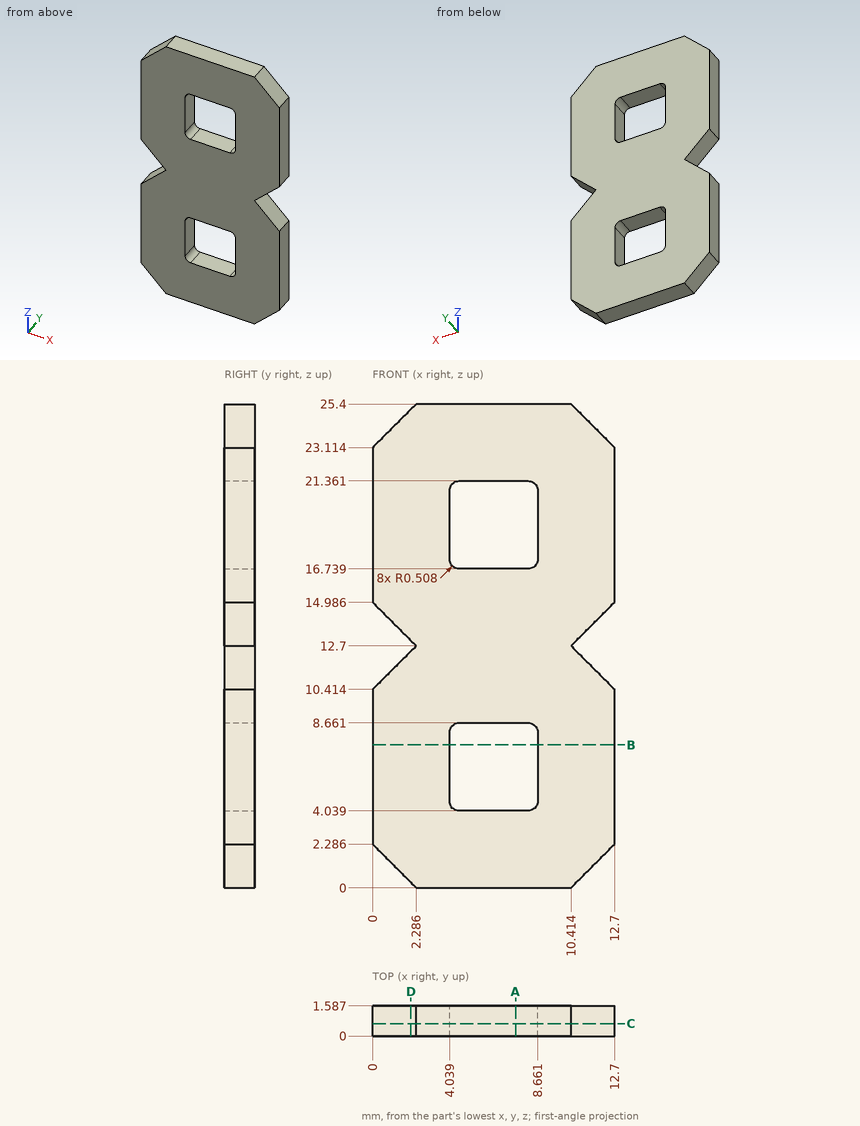
Answer from the drawing. Dimensions are ordinates in mm from the lowest x, y and z of the part. Round coordinates to 2 decimals unless told otherwise and drop trailing zeros. Write each loop counter-clockwise with the first axis right and the second up, starting at its lowest first coordinate (ties: lowest second). Pieces come first, ordered by that corner, then holes.
1. The part is cut by section B-B, the plane z = 7.5. Determine the outline of the cut face in (x, y), then the cut area to 3 significant figures.
2. The part is cut by section C-C, the plane y = 0.65. State how many separate pieces and enclosed holes the cut face has, then the cut area to 3 significant figures.
3. The part is cut by section D-D, the plane x = 2. Determine the outline of the cut face in (y, z) (1 decimal).
4. The part is cut by section A-A, the plane x = 7.5. Determine the outline of the cut face in (y, z).
5. Straight lines are drawn through the part: L1, parallel to Z at x = 7.75, y = 1.4; L2, parallel to X at y = 0.75, z = 7; L3, parallel to Z at x = 12.25, y = 1.1 (1 decimal). For each, find the intervals that lie inside material, in ascending order.
Values:
1. outline: (0, 0) - (4.04, 0) - (4.04, 1.59) - (0, 1.59) - close; (8.66, 0) - (12.7, 0) - (12.7, 1.59) - (8.66, 1.59) - close
1. area: 12.8 mm2
2. separate pieces: 1
2. enclosed holes: 2
2. area: 259 mm2
3. outline: (0, 0.3) - (1.6, 0.3) - (1.6, 12.4) - (0, 12.4) - close; (0, 13) - (1.6, 13) - (1.6, 25.1) - (0, 25.1) - close
4. outline: (0, 0) - (1.59, 0) - (1.59, 4.04) - (0, 4.04) - close; (0, 8.66) - (1.59, 8.66) - (1.59, 16.74) - (0, 16.74) - close; (0, 21.36) - (1.59, 21.36) - (1.59, 25.4) - (0, 25.4) - close
5. L1: z = 0 to 4.04, 8.66 to 16.74, 21.36 to 25.4
5. L2: x = 0 to 4.04, 8.66 to 12.7
5. L3: z = 1.8 to 10.9, 14.5 to 23.6
